Geometry check sheet. Reference: the model listing, model coordinates, mm. Face numbers are marked on the shaded views. A direction names the side the tool comes from. Round coordinates to 2 decimals unless told otherwise and drop trailing zeros. Write each loop counter-clockwise with the first axis right and the second up, starting at its lowest first coordinate (ties: lowest second). Pieces come first, ordered by that corner, then holes. Notation, with made-up numbers: M 61.5,67 L 74.5,67 A23 cw 74.5,99 Z; hole C 11.5,59 d4. An arc over 180 degrees is marked long. Answer in a Markdown table with one row per item. Add a question column.
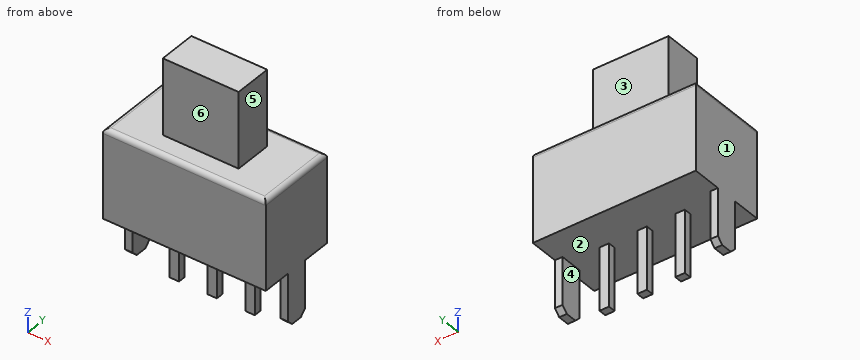
from build123d import *

# Parameters (mm, degrees)
SKETCH1_W           = 8.6
SKETCH1_H           = 4.3
BOSS_EXTRUDE1_DEPTH = 4.7
SKETCH2_W           = 4
SKETCH2_H           = 2
BOSS_EXTRUDE2_DEPTH = 4
SKETCH3_W           = 0.4
SKETCH3_H           = 1.2
BOSS_EXTRUDE3_DEPTH = 2.8
SKETCH4_W           = 0.5
SKETCH4_H           = 0.4
BOSS_EXTRUDE4_DEPTH = 3.3
CHAMFER1_SIZE       = 0.3
FILLET1_R           = 0.25


with BuildPart() as part:
    # Sketch1 → Boss-Extrude1 (new body)
    with BuildSketch(Plane.XY):
        Rectangle(SKETCH1_W, SKETCH1_H)
    extrude(amount=BOSS_EXTRUDE1_DEPTH)

    # Sketch2 → Boss-Extrude2 (add)
    with BuildSketch(Plane.XY.offset(4.7)):
        Rectangle(SKETCH2_W, SKETCH2_H)
    extrude(amount=BOSS_EXTRUDE2_DEPTH)

    # Sketch3 → Boss-Extrude3 (add)
    with BuildSketch(Plane(origin=(0, 0, 0), x_dir=(-1, 0, 0), z_dir=(0, 0, -1))):
        with Locations((-4.1, 0)):
            Rectangle(SKETCH3_W, SKETCH3_H)
        with Locations((4.1, 0)):
            Rectangle(SKETCH3_W, SKETCH3_H)
    extrude(amount=BOSS_EXTRUDE3_DEPTH)

    # Sketch4 → Boss-Extrude4 (add)
    with BuildSketch(Plane(origin=(0, 0, 0), x_dir=(-1, 0, 0), z_dir=(0, 0, -1))):
        with Locations((2, 0)):
            Rectangle(SKETCH4_W, SKETCH4_H)
        Rectangle(SKETCH4_W, SKETCH4_H)
        with Locations((-2, 0)):
            Rectangle(SKETCH4_W, SKETCH4_H)
    extrude(amount=BOSS_EXTRUDE4_DEPTH)

    # Chamfer1
    chamfer1_edges = [part.edges().sort_by_distance(p)[0] for p in [
        (4.1, 0.6, -2.8),
        (4.1, -0.6, -2.8),
        (-4.1, 0.6, -2.8),
        (-4.1, -0.6, -2.8),
    ]]
    chamfer(chamfer1_edges, length=CHAMFER1_SIZE)

    # Fillet1
    fillet1_edges = [part.edges().sort_by_distance(p)[0] for p in [
        (-4.3, 0, 4.7),
        (0, -2.15, 4.7),
        (4.3, 0, 4.7),
        (0, 2.15, 4.7),
    ]]
    fillet(fillet1_edges, radius=FILLET1_R)


solid = part.part
Item 1: Scan lines: probe 1 along X at (y, z) = (-0.5, -0.25); probe 2 along Z at (x, y) = (-2.75, -1.5); probe 3 along Y at (x, z) = (-1.25, 5). Record each from-to range of solid material in increasing order. Write a range as from..to.
Item 2: Access from +Z, -Z, +X, -X, +Y, -Y to the whole of each face (thin tool, end or side, straight path). Record for the marked faces 4, 5 and 6.
Item 3: Section check D-D, the plane z = 6.25. Record the boundary of the cut face in (x, y), and give its area (3 significant figures).
Item 4: Section check B-B, the plane x = -0.5. Record the boundary of the cut face in (y, z).
Item 5: Section check A-A, the plane z = -0.75. Record the boundary of the cut face in (x, y).
Item 6: Section check C-C, the plane y = 1.4. Record the boundary of the cut face in (x, z), and give its area (3 significant figures).
Item 7: Gauge pin test, flat ends, axial feed: pin 1 Ø1.6 at (y, z) = (0, 7.5) entering from -X; pin 2 Ø3 at (x, z) = (0, 6.5) entering from -Y; pin 3 Ø1.2 at (x, z) = (-1, 6) entering from +Y. Record the tip position at first contact, or that the pin passes through.
Item 8: Mould release check, pull along X, two halves, no side actions. Record for the marked faces 1, 2 and 3: +X half, -X half, draft (parallel to the pull), parting line (faces both ways), or undercut.
Result sheet:
| question | item | result |
|---|---|---|
| 1 | probe 1 | x = -4.3..-3.9, 3.9..4.3 |
| 1 | probe 2 | z = 0..4.7 |
| 1 | probe 3 | y = -1..1 |
| 2 | face 4 | -Z, +Y, -Y |
| 2 | face 5 | +Z, +X, +Y, -Y |
| 2 | face 6 | +Z, +X, -X, -Y |
| 3 | outline | M -2,-1 L 2,-1 L 2,1 L -2,1 Z |
| 3 | area | 8.00 mm^2 |
| 4 | outline | M -2.15,0 L 2.15,0 L 2.15,4.45 A0.25 ccw 1.9,4.7 L 1,4.7 L 1,8.7 L -1,8.7 L -1,4.7 L -1.9,4.7 A0.25 ccw -2.15,4.45 Z |
| 5 | outline | M -4.3,-0.6 L -3.9,-0.6 L -3.9,0.6 L -4.3,0.6 Z; M -2.25,-0.2 L -1.75,-0.2 L -1.75,0.2 L -2.25,0.2 Z; M -0.25,-0.2 L 0.25,-0.2 L 0.25,0.2 L -0.25,0.2 Z; M 1.75,-0.2 L 2.25,-0.2 L 2.25,0.2 L 1.75,0.2 Z; M 3.9,-0.6 L 4.3,-0.6 L 4.3,0.6 L 3.9,0.6 Z |
| 6 | outline | M -4.3,0 L 4.3,0 L 4.3,4.45 A0.25 ccw 4.05,4.7 L -4.05,4.7 A0.25 ccw -4.3,4.45 Z |
| 6 | area | 40.4 mm^2 |
| 7 | pin 1 | stops at x = -2 |
| 7 | pin 2 | stops at y = -1 |
| 7 | pin 3 | stops at y = 1 |
| 8 | face 1 | -X half |
| 8 | face 2 | undercut |
| 8 | face 3 | draft |
